Solid Edge part; units mm, degrees
sketch "Sketch1" plane through (0, 0, 0) normal (0, 0, 1) x (1, 0, 0)
  circle A0 centre (0, 0) radius 10.44
extrude "Protrusion1" add sketch "Sketch1" along normal blind 7.76
sketch "Sketch2" plane through (0, 0, 0) normal (0, 0, -1) x (1, 0, 0)
  circle A0 centre (0, 0) radius 6
extrude "Protrusion2" add sketch "Sketch2" along normal blind 45
sketch "Sketch3" plane through (0, 0, -45) normal (0, 0, -1) x (1, 0, 0)
  circle A0 centre (0, 0) radius 5.9997
extrude "Cutout1" cut sketch "Sketch3" against normal blind 30 flip side to cut
chamfer "Chamfer_1" distance 0.9 angle 45 1 edges at (-5.9997, 0, -45)
sketch "Sketch4" plane through (0, 0, 7.76) normal (0, 0, 1) x (1, 0, 0)
  line L0 (-5.2909, 9) -> (5.2909, 9)
extrude "Cutout2" cut sketch "Sketch4" against normal up to next material side at (0, 9.05, 7.76)
pattern_circular "Pattern1" count 6 over 360 about axis through (0, 0, 7.76) along (0, 0, 1) of "Cutout2"
properties part number "119586" material "Steel"
The listing builds one solid part. Answer for the finished solid, in the listing's coordinates (mm). A direction names the side the tool comes from. Coordinates: 2 decimals unless noted, no trailing zeros. Loops run counter-clockwise (first coordinate to the right, second up) from the corner with the lowest first, then second, coordinate; pieces in that order, holes last. Notation, with made-up numbers: (-5.75, -29) -> (51.25, -29) arc R6 cw to (51.25, -24) -> close; hole circle Ø6 at (61.25, 24.25). An arc over 180 degrees is marked (long way). Answer in a Markdown table with one row per item. Add a question column.
1. For faces 1 (the cylindrical face through (5.723, -1.802, -29.754)), 2 (the flat face through (0, 0, -45)), determine the directions among +Z, -Z, +X, -X, +Y, -Y from which every point of the face is accessible in a straight line to the end or side of a thin tool.
2. The part is cut by section C-C, the plane z = -34. Write down the section's boundary in (x, y), then the cut area to 3 significant figures.
3. Flat-ended cylindrical pins translate along their axes: P1, Ø1, axis at x = -6.5, z = 1, coming from the +Y side; P2, Ø8, axis at x = 1, z = -30.5, coming from the -Y side; P3, Ø3, axis at y = -6.5, z = -10.5, coming from the -X side. Find the tip coordinate at first contact, or state that the pin passes through.
4. Consider line 1 (X direction, y = 0, z = -29.5); line 2 (Z direction, x = 8, y = -3.5). Determine where each line is inside the solid, lowest interval first. Write a range as [from, to].
5. The part is cut by section B-B, the plane z = 1. Write down the section's boundary in (x, y).
Answer below:
| question | item | result |
|---|---|---|
| 1 | face 1 | -Z |
| 1 | face 2 | -Z, +X, -X, +Y, -Y |
| 2 | outline | circle Ø12 at (0, 0) |
| 2 | area | 113 mm2 |
| 3 | P1 | y = 7.61 |
| 3 | P2 | y = -6 |
| 3 | P3 | x = -3.32 |
| 4 | line 1 | [-6, 6] |
| 4 | line 2 | [0, 7.76] |
| 5 | outline | (-10.39, 0) -> (-5.2, -9) -> (5.2, -9) -> (10.39, 0) -> (5.2, 9) -> (-5.2, 9) -> close |
